from build123d import *

# Parameters (mm, degrees)
CYLINDER002_R     = 2
CYLINDER002_DEPTH = 4
CYLINDER003_R     = 2
CYLINDER003_DEPTH = 4
BOX001_W          = 4
BOX001_H          = 18
BOX001_DEPTH      = 4


with BuildPart() as cilindro:
    # Cylinder002 → Cylinder002 (new body)
    with BuildSketch(Plane(origin=(0, 11, 1), x_dir=(1, 0, 0), z_dir=(0, 0, 1))):
        Circle(CYLINDER002_R)
    extrude(amount=CYLINDER002_DEPTH)


with BuildPart() as cilindro001:
    # Cylinder003 → Cylinder003 (new body)
    with BuildSketch(Plane(origin=(0, -7, 1), x_dir=(1, 0, 0), z_dir=(0, 0, 1))):
        Circle(CYLINDER003_R)
    extrude(amount=CYLINDER003_DEPTH)


with BuildPart() as fusion:
    # Box001 → Box001 (new body)
    with BuildSketch(Plane(origin=(-2, -7, 1), x_dir=(1, 0, 0), z_dir=(0, 0, 1))):
        with Locations((2, 9)):
            Rectangle(BOX001_W, BOX001_H)
    extrude(amount=BOX001_DEPTH)

    # Fusion: union Cilindro, Cilindro001
    add(cilindro.part)
    add(cilindro001.part)


solid = fusion.part
Geometry check sheet. Reference: the model listing, model coordinates, mm. Give positions to 0.01 mm unless a question says otherwise; leave off trailing zeros. Order: outer loops, then holes, each group sorted by start corner. A loop starts at its lowest first (then second) coordinate and runs counter-clockwise, first axis right, second up.
1) Gauge pin test, flat end, axial feed: pin 1 (1.5 mm diameter, centred on x = 1.5, z = 3.5, fed in from -Y). Record the tip position at first contact, or that the pin passes through.
Results are:
pin 1: stops at y = -8.85
2) Cross-section at A-A (z = 1.35). Record the boundary of the cut face in (x, y), then the cut area to 3 significant figures.
Results are:
outline: (-2, -7) arc R2 ccw to (2, -7) - (2, 11) arc R2 ccw to (-2, 11) - close
area: 84.6 mm2
3) Material ranges on probe 1 along Y at (x, z) = (-1.65, 2.8); probe 2 along Y at (x, z) = (-1.5, 1.9); probe 3 along X at (y, z) = (-7.5, 1.3), recorded low to high.
Results are:
probe 1: y = -8.13 to 12.13
probe 2: y = -8.32 to 12.32
probe 3: x = -1.94 to 1.94
